For this review, take the finished solid that the model builds, in its own axes (mm). Face numbers are marked on the shaded views. Give positions to 0.01 mm unless a question says otherwise; leave off trailing zeros. Write each loop counter-clockwise with the first axis right and the second up, starting at its lowest first coordinate (ties: lowest second). Pieces come first, ordered by that corner, then holes. Notation, with made-up numbers: M 29,61.5 L 38,61.5 A30 ccw 38,97.5 Z; hole C 87.25,18.25 d6. An arc over 180 degrees is marked long. Write item = value, one per line.
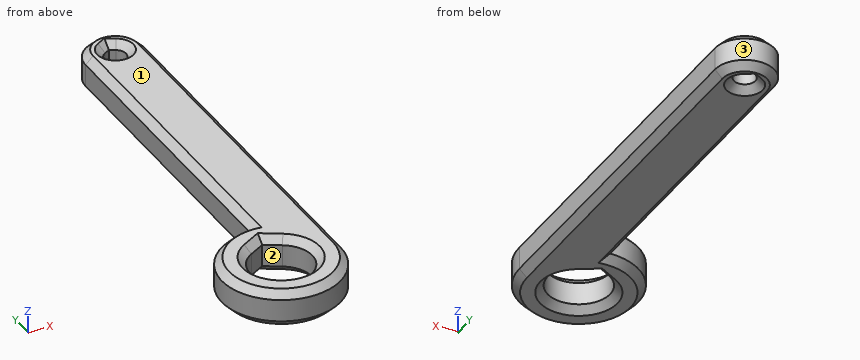
```python
from build123d import *

# Parameters (mm, degrees)
SKETCH_R                   = 8
PAD_DEPTH                  = 5
PAD001_DEPTH               = 5
SKETCH002_R                = 1.45
HOLE_DEPTH                 = 25
HOLE_TEARDROPS_DEPTH       = 25
SKETCH003_R                = 8
PAD002_DEPTH               = 0.9
SKETCH004_R                = 4.2
HOLE001_DEPTH              = 25
HOLE001_TEARDROPS_DEPTH    = 25
HOLE001_TEARDROPS_FACE12_R = 8
POCKET_DEPTH               = 0.9
CHAMFER_SIZE               = 1


with BuildPart() as part:
    # Sketch → Pad (new body)
    with BuildSketch(Plane.XY):
        with Locations((-23, 0)):
            Circle(SKETCH_R)
    extrude(amount=PAD_DEPTH)

    # Sketch001 (on Face3 of Pad) → Pad001 (join)
    with BuildSketch(Plane.XY.offset(5)):
        with BuildLine():
            ThreePointArc((-23, 0), (-19, -4), (-15, 0))
            Line((-15, 0), (-15, 50))
            ThreePointArc((-15, 50), (-19, 54), (-23, 50))
            Line((-23, 0), (-23, 50))
        make_face()
    extrude(amount=-PAD001_DEPTH)

    # Sketch002 (on Face6 of Pad001) → Hole (cut)
    with BuildSketch(Plane.XY.offset(5)):
        with Locations((-19, 50)):
            Circle(SKETCH002_R)
    extrude(amount=-HOLE_DEPTH, mode=Mode.SUBTRACT)

    # Sketch002_Teardrops (on Sketch) → Hole_Teardrops (cut)
    with BuildSketch(Plane.XY.offset(5)):
        with BuildLine():
            ThreePointArc((-19.725, 51.255737), (-19, 48.55), (-18.275, 51.255737))
            Line((-18.275, 51.255737), (-19, 51.674316))
            Line((-19.725, 51.255737), (-19, 51.674316))
        make_face()
    extrude(amount=-HOLE_TEARDROPS_DEPTH, mode=Mode.SUBTRACT)

    # Sketch003 (on Face4 of Hole_Teardrops) → Pad002 (join)
    with BuildSketch(Plane(origin=(0, 0, 0), x_dir=(1, 0, 0), z_dir=(0, 0, -1))):
        with Locations((-23, 0)):
            Circle(SKETCH003_R)
    extrude(amount=PAD002_DEPTH)

    # Sketch004 (on Face2 of Pad002) → Hole001 (cut)
    with BuildSketch(Plane.XY.offset(5)):
        with Locations((-23, 0)):
            Circle(SKETCH004_R)
    extrude(amount=-HOLE001_DEPTH, mode=Mode.SUBTRACT)

    # Sketch004_Teardrops (on Sketch) → Hole001_Teardrops (cut)
    with BuildSketch(Plane.XY.offset(5)):
        with BuildLine():
            ThreePointArc((-25.1, 3.637307), (-23, -4.2), (-20.9, 3.637307))
            Line((-20.9, 3.637307), (-23, 4.849742))
            Line((-25.1, 3.637307), (-23, 4.849742))
        make_face()
    extrude(amount=-HOLE001_TEARDROPS_DEPTH, mode=Mode.SUBTRACT)

    # Hole001_Teardrops Face12 → Pocket (cut)
    with BuildSketch(Plane(origin=(-23, -0.028446, -0.9), x_dir=(0, -1, 0), z_dir=(0, 0, -1))):
        with Locations((-0.028446, 0)):
            Circle(HOLE001_TEARDROPS_FACE12_R)
        with BuildLine():
            ThreePointArc((-0.028446, -4.2), (-2.128446, -3.637307), (-3.665753, -2.1))
            Line((-3.665753, -2.1), (-4.878188, 0))
            Line((-4.878188, 0), (-3.665753, 2.1))
            ThreePointArc((-3.665753, 2.1), (3.608861, 2.1), (-0.028446, -4.2))
        make_face(mode=Mode.SUBTRACT)
    extrude(amount=-POCKET_DEPTH, mode=Mode.SUBTRACT)

    # Chamfer
    chamfer_edges = [part.edges().sort_by_distance(p)[0] for p in [
        (-19.725, 48.744263, 0),
        (-23, 29, 0),
        (-23, 29, 5),
        (-25.1, -3.637307, 0),
        (-25.1, -3.637307, 5),
        (-19.725, 48.744263, 5),
    ]]
    chamfer(chamfer_edges, length=CHAMFER_SIZE)


solid = part.part
```
1. Insertion check: P1, Ø1, axis at x = -27.5, z = 2.5, coming from the -Y side; P2, Ø2, axis at x = -29, z = 2, coming from the +Y side (3 decimals); P3, Ø2.5, axis at y = 36.5, z = 3, coming from the -X side. Each pin has a flat end and moves straight along its axis. Give the tip position at first contact, or say it passes through.
Responses:
P1 = -6.93
P2 = 6.245
P3 = -23
2. We need section B-B, the plane y = 40.5. Write out the cut boundary in (x, z), then the cut area to 3 significant figures.
Responses:
outline = M -23,1 L -22,0 L -16,0 L -15,1 L -15,4 L -16,5 L -22,5 L -23,4 Z
area = 38.0 mm2
3. For line 1 along X through (y, z) = (15, 2.8); line 2 along Y through (x, z) = (-19.25, 2.2); line 3 along X through (y, z) = (4, 3.1), list the stretches that pass through material, from the lowest coordinate up. Write a range as from..to.
Responses:
line_1 = -23..-15
line_2 = -7.07..-1.89, 1.89..48.57, 51.53..53.99
line_3 = -29.93..-24.47, -21.53..-15
4. The part is to be moulded in two halves that separate along Y. For the marked faces 1, 2 and 3, say which applies: +Y half, -Y half, draft (parallel to the pull), parting line (faces both ways), or undercut.
Responses:
face_1 = draft
face_2 = undercut
face_3 = +Y half
5. We need section A-A, the plane z = 2.4. Write out the cut boundary in (x, y) (3 decimals), then the cut area to 3 significant figures.
Responses:
outline = M -23,8 A8 ccw long -15,0 L -15,50 A4 ccw -23,50 Z; hole M -25.1,3.637 A4.2 ccw long -20.9,3.637 L -23,4.85 Z; hole M -19.725,51.256 A1.45 ccw long -18.275,51.256 L -19,51.674 Z
area = 513 mm2
